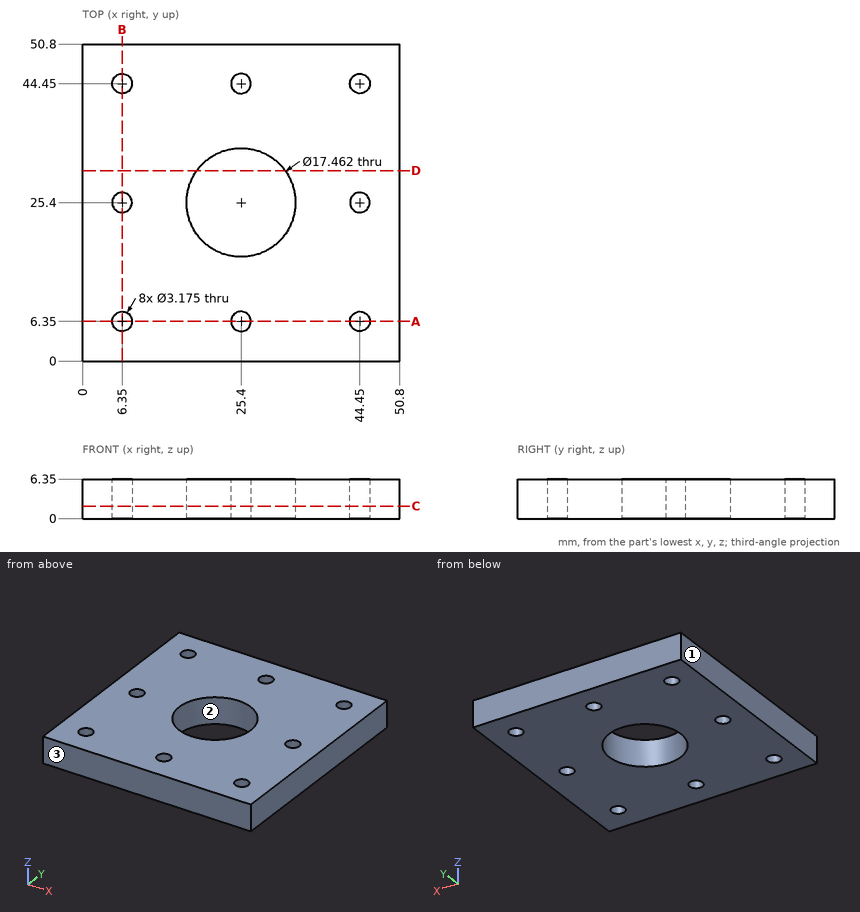
Here's the drawing with two shaded views (mm, measured from the low corner). I have some questions. Give positions to 0.01 mm unless a question says otherwise; leave off trailing zeros. Order: outer loops, then holes, each group sorted by start corner. A loop starts at its lowest first (then second) coordinate and runs counter-clockwise, first axis right, second up. Notation, with made-up numbers: M 52,53 L 80,53 A13 ccw 80,74 Z; hole C 9.25,-28 d7. An arc over 180 degrees is marked long. Answer as a JSON object with one key per item and string values. Group by question number.
1) Suppose I cut it at A-A, the plane y = 6.35. Write out the boundary of the cut face in (x, z), plus the area to 3 significant figures.
2) Suppose I cut it at C-C, the plane z = 2. Count the separate pieces of the cut face and the enclosed holes in it, plus the area to 3 significant figures.
3) Please list where these lines run through material, in increasing order: L1, parallel to Y at x = 25.4, z = 4.25; L2, parallel to Y at x = 44.45, z = 2.5; L3, parallel to X at y = 29, z = 4.75 (1 decimal). Write a range as [from, to].
4) We'd pull the mould along Y, two halves only. Please class the marked faces 1, 2 and 3: pulls with the +Y half, pulls with the -Y half, needs draft (parallel to the pull), parting line crosses it, or undercut.
5) Suppose I cut it at D-D, the plane y = 30.5. Write out the boundary of the cut face in (x, z).
Results found:
{
 "1": {"outline": "M 0,0 L 4.76,0 L 4.76,6.35 L 0,6.35 Z; M 7.94,0 L 23.81,0 L 23.81,6.35 L 7.94,6.35 Z; M 26.99,0 L 42.86,0 L 42.86,6.35 L 26.99,6.35 Z; M 46.04,0 L 50.8,0 L 50.8,6.35 L 46.04,6.35 Z", "area": "262 mm²"},
 "2": {"separate pieces": "1", "enclosed holes": "9", "area": "2,280 mm²"},
 "3": {"L1": "[0, 4.76], [7.94, 16.67], [34.13, 42.86], [46.04, 50.8]", "L2": "[0, 4.76], [7.94, 23.81], [26.99, 42.86], [46.04, 50.8]", "L3": "[0, 17.4], [33.4, 50.8]"},
 "4": {"face 1": "needs draft", "face 2": "undercut", "face 3": "pulls with the -Y half"},
 "5": {"outline": "M 0,0 L 18.31,0 L 18.31,6.35 L 0,6.35 Z; M 32.49,0 L 50.8,0 L 50.8,6.35 L 32.49,6.35 Z"}
}
